Autodesk Inventor part; units mm, degrees
ref_plane "YZ Plane" through (0, 0, 0) normal (1, 0, 0) x (0, 1, 0)
ref_plane "XZ Plane" through (0, 0, 0) normal (0, 1, 0) x (-1, 0, 0)
ref_plane "XY Plane" through (0, 0, 0) normal (0, 0, 1) x (1, 0, 0)
sketch "Эскиз1" plane through (0, 0, 0) normal (0, 1, 0) x (-1, 0, 0)
  line L0 (0, 0) -> (120, 0)
  line L1 (120, 0) -> (120, -120)
  line L2 (120, -120) -> (0, -120)
  line L3 (0, -120) -> (0, 0)
  dimension "d0" = 120
  dimension "d1" = 120
sketch "Эскиз2" plane through (0, 0, 0) normal (0, 1, 0) x (-1, 0, 0)
  circle A0 centre (60, -60) radius 45
  point P0 (0, 0)
  dimension "d2" = 90
  dimension "d3" = 60
  dimension "d4" = 60
extrude "Выдавливание1" add sketch "Эскиз1" along normal blind 16
fillet "Сопряжение1" radius 3 4 edges at (-120, 8, 0) (0, 8, 0) (0, 8, -120) (-120, 8, -120)
extrude "Выдавливание2" cut sketch "Эскиз2" along normal blind 16
sketch "Эскиз3" plane through (0, 16, 0) normal (0, 1, 0) x (1, 0, 0)
  circle A0 centre (-112.5, 7.5) radius 2.5
  circle A1 centre (-7.5, 7.5) radius 2.5
  circle A2 centre (-7.5, 112.5) radius 2.5
  circle A3 centre (-112.5, 112.5) radius 2.5
  line L0 (0, 3) -> (0, 117)
  point P0 (0, 0)
  dimension "d10" = 5
  dimension "d11" = 5
  dimension "d12" = 5
  dimension "d13" = 5
  dimension "d14" = 112.5
  dimension "d15" = 7.5
  dimension "d16" = 7.5
  dimension "d17" = 7.5
  dimension "d18" = 105
  dimension "d19" = 7.5
  dimension "d20" = 105
  dimension "d21" = 105
extrude "Выдавливание3" cut sketch "Эскиз3" against normal blind 16
properties part number "NoctuaNF-A12x15"
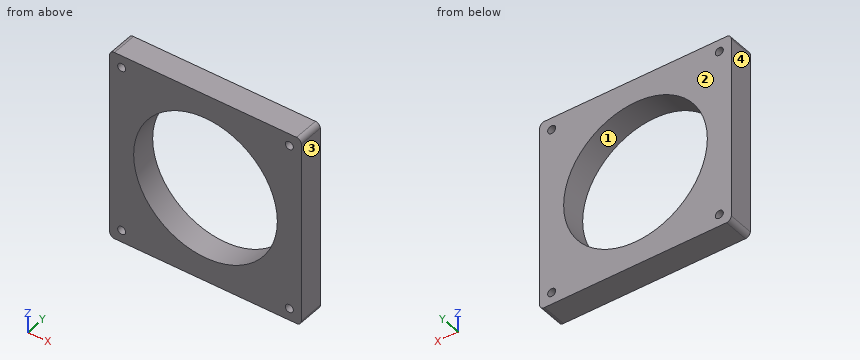
Check sheet for the modelled part. Datum: model origin and axes. Units: mm. Face numbers are marked on the shaded views. Round coordinates to 2 decimals unless told otherwise and drop trailing zeros. Order: outer loops, then holes, each group sorted by start corner. A loop starts at its lowest first (then second) coordinate and runs counter-clockwise, first axis right, second up. Notation, with made-up numbers: (74, 17) - (78, 17) arc R25 ccw to (78, 54) - close; hole circle Ø10 at (87, 10). An arc over 180 degrees is marked (long way). Write item = value, one per line.
Q1. Draft check along X on the marked faces 1, 2, 3 and 4. Enter one of: pulls with the +X half, pulls with the -X half, needs draft (parallel to the pull), parting line crosses it, or undercut.
Computed:
face_1 = undercut
face_2 = needs draft
face_3 = pulls with the +X half
face_4 = pulls with the -X half
Q2. Section check B-B (x = -7.5). Record the boundary of the cut face in (y, z).
Computed:
outline = (0, -120) - (16, -120) - (16, -115) - (0, -115) - close; (0, -110) - (16, -110) - (16, -10) - (0, -10) - close; (0, -5) - (16, -5) - (16, 0) - (0, 0) - close
Q3. Section check A-A (z = -7.5). Record the boundary of the cut face in (x, y), and give its area (3 significant figures).
Computed:
outline = (-120, 0) - (-115, 0) - (-115, 16) - (-120, 16) - close; (-110, 0) - (-10, 0) - (-10, 16) - (-110, 16) - close; (-5, 0) - (0, 0) - (0, 16) - (-5, 16) - close
area = 1,760 mm^2
Q4. Thickness scan on line 1 along Z through (x, y) = (-7.5, 12); line 2 along X through (y, z) = (8, -114). Record the ranges inside material, lowest first.
Computed:
line_1 = -120 to -115, -110 to -10, -5 to 0
line_2 = -120 to -114.5, -110.5 to -9.5, -5.5 to 0
Q5. Section check D-D (z = -60). Record the boundary of the cut face in (x, y), and give its area (3 significant figures).
Computed:
outline = (-120, 0) - (-105, 0) - (-105, 16) - (-120, 16) - close; (-15, 0) - (0, 0) - (0, 16) - (-15, 16) - close
area = 480 mm^2
Q6. Section check C-C (y = 7.75). Record the boundary of the cut face in (x, z), and give its area (3 significant figures).
Computed:
outline = (-120, -117) arc R3 ccw to (-117, -120) - (-3, -120) arc R3 ccw to (0, -117) - (0, -3) arc R3 ccw to (-3, 0) - (-117, 0) arc R3 ccw to (-120, -3) - close; hole circle Ø5 at (-112.5, -112.5); hole circle Ø5 at (-112.5, -7.5); hole circle Ø90 at (-60, -60); hole circle Ø5 at (-7.5, -112.5); hole circle Ø5 at (-7.5, -7.5)
area = 7,950 mm^2
